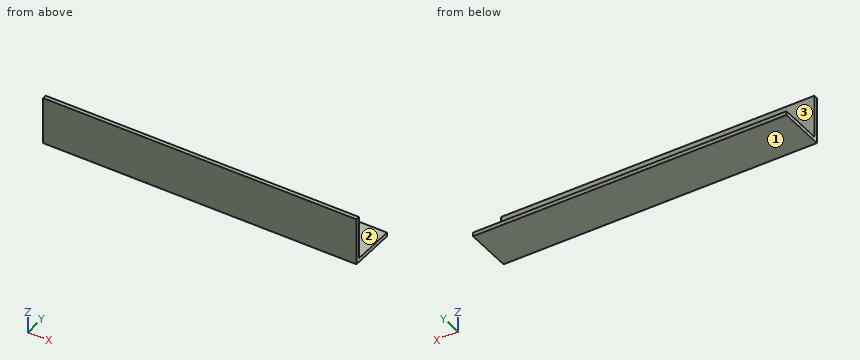
Autodesk Inventor part; units mm, degrees
ref_plane "YZ Plane" through (0, 0, 0) normal (1, 0, 0) x (0, 1, 0)
ref_plane "XZ Plane" through (0, 0, 0) normal (0, 1, 0) x (-1, 0, 0)
ref_plane "XY Plane" through (0, 0, 0) normal (0, 0, 1) x (1, 0, 0)
sketch "Sketch1" plane through (0, 0, 0) normal (0, 0, 1) x (1, 0, 0)
  line L0 (0, 0) -> (254, 0)
  line L1 (254, 0) -> (254, 38.1)
  line L2 (254, 38.1) -> (0, 38.1)
  line L3 (0, 38.1) -> (0, 0)
  dimension "d0" = 254
  dimension "d1" = 38.1
extrude "Extrusion1" add sketch "Sketch1" along normal blind 3.175
sketch "Sketch2" plane through (0, 0, 3.175) normal (0, 0, 1) x (1, 0, 0)
  line L0 (0, 0) -> (254, 0)
  line L1 (0, 0) -> (254, 0)
  line L2 (254, 0) -> (254, 3.175)
  line L3 (254, 3.175) -> (0, 3.175)
  line L4 (0, 3.175) -> (0, 0)
  dimension "d4" = 3.175
  dimension "d5" = 254
extrude "Extrusion2" add sketch "Sketch2" along normal blind 34.925
properties part number "CLB_061_OutsideLBracket"
The model under review builds one solid part; all positions refer to its coordinate system, in mm. Face numbers are marked on the shaded views. Coordinates: 2 decimals unless noted, no trailing zeros. Order: outer loops, then holes, each group sorted by start corner. A loop starts at its lowest first (then second) coordinate and runs counter-clockwise, first axis right, second up. Notation, with made-up numbers: (2, -9) -> (15, -9) arc R13 ccw to (15, 6) -> close; hole circle Ø7 at (51.5, -33.75). An arc over 180 degrees is marked (long way). Answer in a Markdown table with one row per item. Add a question column.
Item 1: Clearance check with flat-ended pins moving along their axes: pin 1 (10 mm diameter, centred on y = 17.5, z = 9, fed in from -X); pin 2 (17.5 mm diameter, centred on x = 133, y = 12.5, fed in from +Z) (3 decimals); pin 3 (10.5 mm diameter, centred on x = 73.5, z = 28, fed in from +Y) (3 decimals). State where each tip first meets the part, or that it passes through.
Item 2: To check wall thickness, follow probe 1 along Z at (x, y) = (232.5, 25.5) (3 decimals). State the ranges of the line that lie inside material, in increasing order.
Item 3: Mouldability with a two-part tool opening along Z and no side actions: class the marked faces 1, 2 and 3 as +Z half, -Z half, draft (parallel to the pull), parting line (faces both ways), or undercut.
Item 4: We need section B-B on z = 35. Write out the cut boundary in (x, y) (3 decimals).
Item 5: We need section A-A on x = 158. Write out the cut boundary in (y, z) (3 decimals), plus the area to 3 significant figures.
Final values:
| question | item | result |
|---|---|---|
| 1 | pin 1 | passes through |
| 1 | pin 2 | stops at z = 3.175 |
| 1 | pin 3 | stops at y = 3.175 |
| 2 | probe 1 | z = 0 to 3.175 |
| 3 | face 1 | -Z half |
| 3 | face 2 | +Z half |
| 3 | face 3 | draft |
| 4 | outline | (0, 0) -> (254, 0) -> (254, 3.175) -> (0, 3.175) -> close |
| 5 | outline | (0, 0) -> (38.1, 0) -> (38.1, 3.175) -> (3.175, 3.175) -> (3.175, 38.1) -> (0, 38.1) -> close |
| 5 | area | 232 mm2 |
